Geometry: see drawing. Coordinates: mm, zero at the bounding-box minimum. A direction names the side the tool comes from. Coordinates: 2 decimals unless noted, no trailing zeros. Write each loop counter-clockwise with the first axis right and the second up, starting at its lowest first coordinate (ties: lowest second). Pieces come first, ordered by that corner, then holes.
1) Line query: L1, parallel to X at y = 9, z = 14.5; L2, parallel to Z at x = 25, y = 20.5. Output: solid intervals per line, ascending.
2) Section query A-A (x = 27.5). Output: boundary loops of the cut face in (y, z), then the cut area to 3 significant figures.
3) Section query D-D (x = 8). Output: boundary loops of the cut face in (y, z), then the cut area to 3 significant figures.
4) Pin query (flat end, axial travel): pin 1 Ø5 at (y, z) = (12, 26.5) entering from +X; pin 2 Ø8 at (x, z) = (24.5, 22.5) entering from -Y; pin 3 Ø9.5 at (x, z) = (20.5, 23.5) entering from +Y. Return the tip coordinate at first contact, or that it passes through.
5) Set-up query: the marked faces 1, 2 and 3. Return all of +Z, -Z, +X, -X, +Y, -Y with unobstructed straight access to the full face (end or side cutting, diameter ignored); none if empty.
6) Section query B-B (z = 19). Output: boundary loops of the cut face in (x, y).
7) Section query C-C (y = 15). Output: boundary loops of the cut face in (x, z).
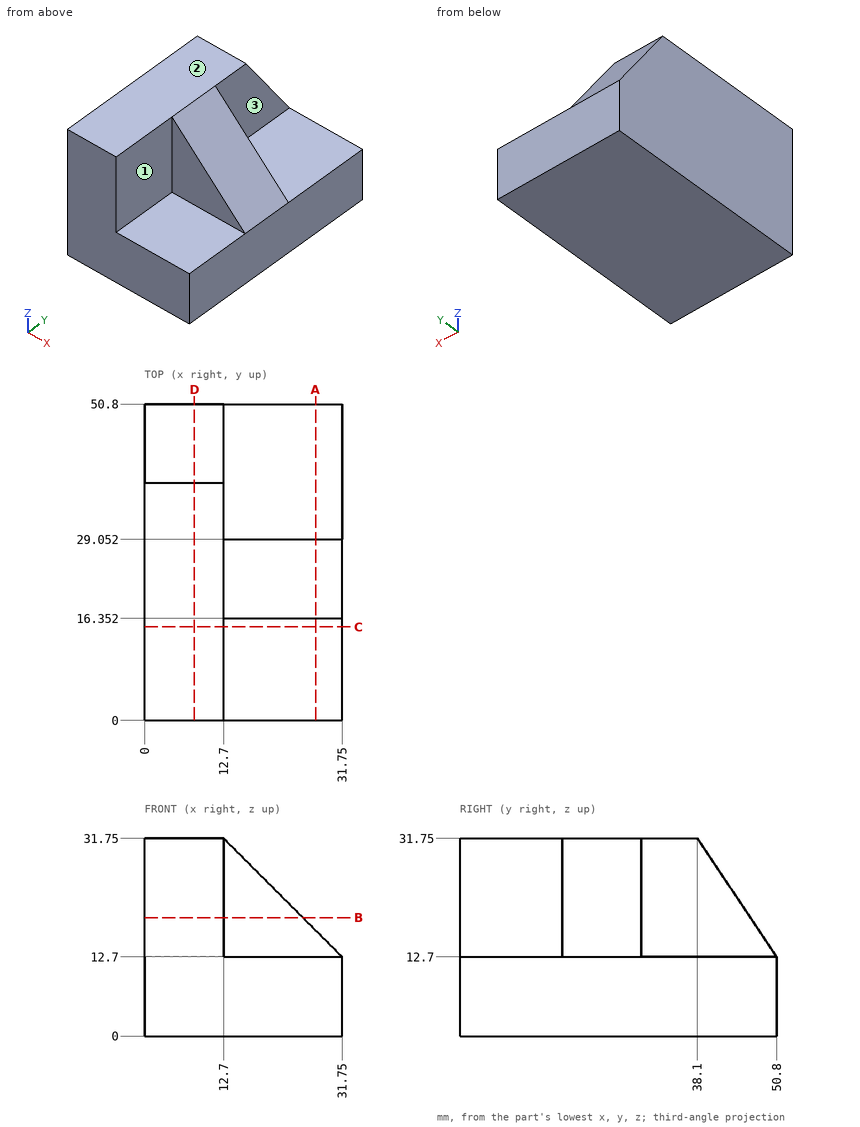
Answer:
1. L1: x = 0 to 12.7
1. L2: z = 0 to 19.45
2. outline: (0, 0) - (50.8, 0) - (50.8, 12.7) - (29.05, 12.7) - (29.05, 16.95) - (16.35, 16.95) - (16.35, 12.7) - (0, 12.7) - close
2. area: 699 mm2
3. outline: (0, 0) - (50.8, 0) - (50.8, 12.7) - (38.1, 31.75) - (0, 31.75) - close
3. area: 1,490 mm2
4. pin 1: stops at x = 12.7
4. pin 2: stops at y = 16.35
4. pin 3: stops at y = 29.05
5. face 1: +Z, +X, -Y
5. face 2: +Z, +X, -X, +Y, -Y
5. face 3: +Z, +X, +Y
6. outline: (0, 0) - (12.7, 0) - (12.7, 16.35) - (25.45, 16.35) - (25.45, 29.05) - (12.7, 29.05) - (12.7, 46.6) - (0, 46.6) - close
7. outline: (0, 0) - (31.75, 0) - (31.75, 12.7) - (12.7, 12.7) - (12.7, 31.75) - (0, 31.75) - close
